Could you check a few things on this model? Use its own coordinates, in mm. A direction names the side the tool comes from. Give positions to 0.01 mm unless a question says otherwise; leave off trailing zeros. Write each loop counter-clockwise with the first axis right and the second up, starting at its lowest first coordinate (ties: lowest second). Pieces come first, ordered by that corner, then holes. Notation, with made-up numbers: (38.25, 19) - (85.25, 19) arc R18 ccw to (85.25, 50) - close; hole circle Ø4 at (64, 77.25). An arc over 180 degrees is marked (long way). Use one line per item in the form item = value.
Autodesk Inventor part; units mm, degrees
ref_plane "YZ Plane" through (0, 0, 0) normal (1, 0, 0) x (0, 1, 0)
ref_plane "XZ Plane" through (0, 0, 0) normal (0, 1, 0) x (-1, 0, 0)
ref_plane "XY Plane" through (0, 0, 0) normal (0, 0, 1) x (1, 0, 0)
sketch "Sketch1" plane through (0, 0, 0) normal (0, 0, 1) x (1, 0, 0)
  line L0 (-25.5474, 19.5864) -> (55.7326, 19.5864)
  line L1 (55.7326, 19.5864) -> (55.7326, -101.0636)
  line L2 (55.7326, -101.0636) -> (-25.5474, -101.0636)
  line L3 (-25.5474, -101.0636) -> (-25.5474, 19.5864)
  dimension "d0" = 81.28
  dimension "d1" = 120.65
extrude "Extrusion1" add sketch "Sketch1" along normal blind 5.08
sketch "Sketch2" plane through (0, 0, 5.08) normal (0, 0, 1) x (1, 0, 0)
  line L0 (55.7326, 19.5864) -> (55.7326, -101.0636)
  line L1 (-25.5474, 19.5864) -> (55.7326, 19.5864)
  line L2 (-25.5474, -101.0636) -> (-25.5474, 19.5864)
  line L3 (55.7326, -101.0636) -> (-25.5474, -101.0636)
  line L4 (-19.1974, 4.3464) -> (49.3826, 4.3464)
  line L5 (49.3826, 4.3464) -> (43.6676, -61.6936)
  line L6 (43.6676, -61.6936) -> (-13.4824, -61.6936)
  line L7 (-13.4824, -61.6936) -> (-19.1974, 4.3464)
  circle A0 centre (15.0926, 4.3464) radius 40.64 construction
  circle A1 centre (15.0926, 4.3464) radius 34.29 construction
  circle A2 centre (15.0926, -61.6936) radius 28.575 construction
  dimension "d4" = 57.15
  dimension "d5" = 68.58
  dimension "d6" = 15.24
  dimension "d7" = 66.04
hole "Hole1" at (-19.1974, 4.3464, 5.08) at (49.3826, 4.3464, 5.08) at (43.6676, -61.6936, 5.08) at (-13.4824, -61.6936, 5.08) direction (0, 0, -1) diameter 3.175 end through all
sketch "Sketch3" plane through (-25.5474, 19.5864, 0) normal (0, 1, 0) x (1, 0, 0)
  line L0 (0, -5.08) -> (81.28, -5.08)
  line L1 (81.28, 0) -> (81.28, -5.08)
  line L2 (0, 0) -> (81.28, 0)
  line L3 (0, 0) -> (0, -5.08)
sketch "Sketch4" plane through (-25.5474, 19.5864, 0) normal (0, 1, 0) x (1, 0, 0)
  line L0 (81.28, 0) -> (81.28, -5.08)
  line L1 (0, 0) -> (81.28, 0)
  line L2 (0, 0) -> (0, -5.08)
  line L3 (39.37, 0) -> (41.91, 0)
  line L4 (41.91, 0) -> (41.91, 1.27)
  line L5 (41.91, 1.27) -> (39.37, 1.27)
  line L6 (39.37, 1.27) -> (39.37, 0)
  circle A0 centre (40.64, 0.4048) radius 1.27 construction
  circle A1 centre (40.64, 0.4048) radius 40.64 construction
  dimension "d15" = 2.54
  dimension "d16" = 1.27
extrude "Extrusion2" add sketch "Sketch4" against normal blind 12.7
sketch "Sketch5" plane through (-25.5474, 6.8864, 0) normal (0, -1, 0) x (1, 0, 0)
  line L0 (41.91, 0) -> (41.91, -1.27)
  line L1 (39.37, 0) -> (41.91, 0)
  line L2 (39.37, -1.27) -> (39.37, 0)
  line L3 (41.91, -1.27) -> (39.37, -1.27)
  line L4 (27.94, 0) -> (53.34, 0)
  line L5 (53.34, 0) -> (53.34, -1.27)
  line L6 (53.34, -1.27) -> (27.94, -1.27)
  line L7 (27.94, -1.27) -> (27.94, 0)
  circle A0 centre (40.64, -8.0178) radius 1.27 construction
  circle A1 centre (40.64, -8.0178) radius 12.7 construction
  dimension "d19" = 25.4
extrude "Extrusion3" add sketch "Sketch5" against normal blind 2.54
sketch "Sketch7" plane through (0, 0, 0) normal (0, 0, -1) x (-1, 0, 0)
  line L0 (-55.7326, 19.5864) -> (-55.7326, -101.0636)
  line L1 (25.5474, -101.0636) -> (25.5474, 19.5864)
  circle A0 centre (13.4824, -61.6936) radius 1.5875
  circle A1 centre (-5.5676, -86.3316) radius 5.08
  circle A2 centre (-5.5676, -86.3316) radius 1.905
  circle A3 centre (-24.6176, -86.3316) radius 5.08
  circle A4 centre (-24.6176, -86.3316) radius 1.905
  circle A5 centre (-15.0926, -74.2033) radius 15.4215 construction
  circle A6 centre (-15.0926, -74.2033) radius 40.64 construction
  dimension "d26" = 19.05
  dimension "d27" = 24.638
  dimension "d28" = 3.81
  dimension "d29" = 10.16
extrude "Extrusion5" add sketch "Sketch7" along normal blind 7.62 contours A1 | A3
properties part number "baseplate"
1. For pin 1 (1.1 mm diameter, centred on x = 5.5, y = -86, fed in from -Z); pin 2 (0.6 mm diameter, centred on x = 10.5, z = -1, fed in from +Y); pin 3 (10 mm diameter, centred on x = 13.5, y = 11, fed in from -Z), each with a flat end and sliding along its axis, tell me the tip position at first contact or that it passes through.
Response values:
pin_1 = 0
pin_2 = 9.43
pin_3 = -1.27
2. If we mould it in two halves opening along X, with no side actions, what happens to faces 1 (the face through (22, -86, -7.62)), 2 (the face through (6, -86, 0)), 3 (the face through (55.733, -40, 3))? For each: pulls with the +X half, pulls with the -X half, needs draft (parallel to the pull), parting line crosses it, or undercut.
Response values:
face_1 = needs draft
face_2 = undercut
face_3 = pulls with the +X half
3. Imagine slicing it at B-B, the plane y = 4. List the corners of the cut face in (x, z) for me, and give its area (3 significant figures).
Response values:
outline = (-25.55, 0) - (-20.75, 0) - (-20.75, 5.08) - (-25.55, 5.08) - close; (-17.65, 0) - (47.83, 0) - (47.83, 5.08) - (-17.65, 5.08) - close; (50.93, 0) - (55.73, 0) - (55.73, 5.08) - (50.93, 5.08) - close
area = 381 mm²
4. Imagine slicing it at A-A, the plane z = -3.25. List the corners of the cut face in (x, y) for me (3 decimals), and give its area (3 significant figures).
Response values:
outline = circle Ø10.16 at (5.568, -86.332); circle Ø10.16 at (24.618, -86.332); hole circle Ø3.81 at (5.568, -86.332); hole circle Ø3.81 at (24.618, -86.332)
area = 139 mm²
5. Which directions (+Z, -Z, +X, -X, +Y, -Y) give clear straight access to the entire face, cutting with the end or side of a thin tool? Please do faces 4 (the face through (-17.648, 4.691, 2.504)), 5 (the face through (0.875, -84.386, -3.757)), 6 (the face through (15, 10, -1.27)).
Response values:
face_4 = +Z, -Z
face_5 = -Z
face_6 = -Z, +X, -X, +Y
6. If I drill on line 1 (Y direction, x = 5.5, z = -3.25); line 2 (Z direction, x = -18, y = -33); line 3 (X direction, y = -87, z = -2), over which ranges is the centre line in solid material (lowest first)? Write a range as from..to.
Response values:
line_1 = -91.41..-88.24, -84.43..-81.25
line_2 = 0..5.08
line_3 = 0.53..3.78, 7.35..10.6, 19.58..22.83, 26.4..29.65
7. Imagine slicing it at C-C, the plane y = -36. List the corners of the cut face in (x, z) for me, and give its area (3 significant figures).
Response values:
outline = (-25.55, 0) - (55.73, 0) - (55.73, 5.08) - (-25.55, 5.08) - close
area = 413 mm²
